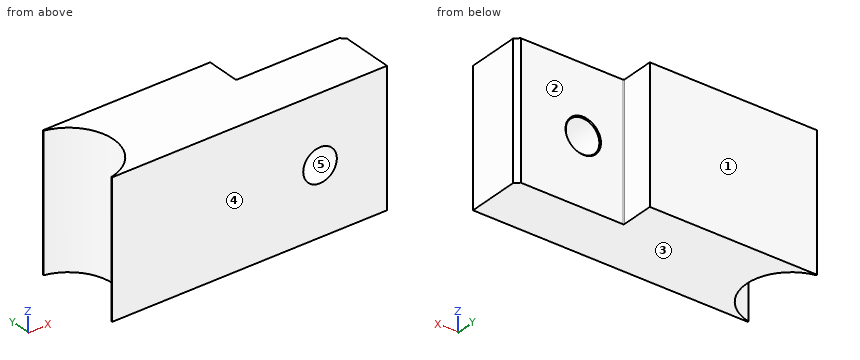
from build123d import *

# Parameters (mm, degrees)
BOSS_EXTRUDE1_DEPTH          = 38.1
F_3_8_0_375_DIAMETER_HOLE1_D = 9.525
CHAMFER1_SIZE                = 1.27
CHAMFER2_SIZE                = 0.254
FILLET1_R                    = 0.254


with BuildPart() as part:
    # Sketch1 → Boss-Extrude1 (new body)
    with BuildSketch(Plane.XY):
        with BuildLine():
            Line((2.54, 0), (80.402581892, 0))
            Line((80.402581892, 0), (80.402581892, 15.875))
            Line((80.402581892, 15.875), (49.922581892, 15.875))
            Line((49.922581892, 15.875), (49.922581892, 25.4))
            Line((49.922581892, 25.4), (2.54, 25.4))
            Line((2.54, 25.4), (2.54, 25.143407893))
            ThreePointArc((2.54, 25.143407893), (12.7, 12.7), (2.54, 0.256592107))
            Line((2.54, 0.256592107), (2.54, 0))
        make_face()
    extrude(amount=BOSS_EXTRUDE1_DEPTH)

    # 3/8 (0.375) Diameter Hole1 (through all)
    with Locations(Plane(origin=(0, 15.875, 0), x_dir=(1, 0, 0), z_dir=(0, 1, 0))):
        with Locations((61.425582, -19.05)):
            Hole(F_3_8_0_375_DIAMETER_HOLE1_D / 2)

    # Chamfer1
    chamfer1_edges = [part.edges().sort_by_distance(p)[0] for p in [
        (80.402581892, 15.875, 19.05),
    ]]
    chamfer(chamfer1_edges, length=CHAMFER1_SIZE)

    # Chamfer2
    chamfer2_edges = [part.edges().sort_by_distance(p)[0] for p in [
        (66.188082, 15.875, 19.05),
    ]]
    chamfer(chamfer2_edges, length=CHAMFER2_SIZE)

    # Fillet1
    fillet1_edges = [part.edges().sort_by_distance(p)[0] for p in [
        (49.922581892, 15.875, 19.05),
    ]]
    fillet(fillet1_edges, radius=FILLET1_R)


solid = part.part
Could you check a few things on this model? Use its own coordinates, in mm. Face numbers are marked on the shaded views. A direction names the side the tool comes from. Give positions to 0.01 mm unless a question says otherwise; leave off trailing zeros. Order: outer loops, then holes, each group sorted by start corner. A loop starts at its lowest first (then second) coordinate and runs counter-clockwise, first axis right, second up. Notation, with made-up numbers: M 13.5,81 L 31.5,81 A26 cw 31.5,118 Z; hole C -35.5,65 d3. An arc over 180 degrees is marked long. One line per question, with ' | ' between items.
1. We'd pull the mould along Z, two halves only. Please class the marked faces 3, 4 and 5: +Z half, -Z half, draft (parallel to the pull), parting line (faces both ways), or undercut.
Results:
face 3: -Z half | face 4: draft | face 5: undercut
2. I'm going to push flat-ended pins straight in: pin 1 (1 mm diameter, centred on x = 62, z = 25.5, fed in from +Y) (3 decimals); pin 2 (3 mm diameter, centred on y = 18, z = 24.5, fed in from +X); pin 3 (8.5 mm diameter, centred on x = 61.43, z = 19.05, fed in from +Y). Where does each tip first touch, or does it pass through?
Results:
pin 1: y = 15.875 | pin 2: x = 49.92 | pin 3: through
3. I want a section at A-A (z = 19.05). List the corners of the cut face in (x, y) for me (3 decimals), and give its area (3 significant figures).
Results:
outline: M 2.54,0 L 56.663,0 L 56.663,15.621 L 56.409,15.875 L 50.177,15.875 A0.254 cw 49.923,16.129 L 49.923,25.4 L 2.54,25.4 L 2.54,25.143 A12.7 cw 2.54,0.257 Z; M 66.188,0 L 80.403,0 L 80.403,14.605 L 79.133,15.875 L 66.442,15.875 L 66.188,15.621 Z | area: 1,350 mm²
4. If I drill on line 1 (Y direction, x = 65.5, z = 10) (3 decimals); line 2 (X direction, y = 7.75, z = 19.05); line 3 (X direction, y = 14.75, z = 33), over which ranges is the centre line in solid material (lowest first)?
Results:
line 1: 0 to 15.875 | line 2: 11.7 to 56.66, 66.19 to 80.4 | line 3: 12.53 to 80.26
5. I want a section at D-D (x = 54.5). List the corners of the cut face in (y, z) for me (3 decimals), and give its area (3 significant figures).
Results:
outline: M 0,0 L 15.875,0 L 15.875,38.1 L 0,38.1 Z | area: 605 mm²
6. For the marked faces 1 and 2, which set-ups out of +Z, -Z, +X, -X, +Y, -Y let a thin tool reach every point of the face, with its end or its side?
Results:
face 1: +Z, -Z, +X, -X, +Y | face 2: +Z, -Z, +X, +Y
7. I want a section at B-B (z = 10). List the corners of the cut face in (x, y) for me (3 decimals), and give its area (3 significant figures).
Results:
outline: M 2.54,0 L 80.403,0 L 80.403,14.605 L 79.133,15.875 L 50.177,15.875 A0.254 cw 49.923,16.129 L 49.923,25.4 L 2.54,25.4 L 2.54,25.143 A12.7 cw 2.54,0.257 Z | area: 1,500 mm²
